from build123d import *

# Parameters (mm, degrees)
SKETCH1_W                  = 650
SKETCH1_H                  = 160
BOSS_EXTRUDE1_DEPTH        = 20
FILLET1_R                  = 10
F_11_0_11_DIAMETER_HOLE1_D = 11
F_7_0_7_DIAMETER_HOLE1_D   = 7
F_4_0_4_DIAMETER_HOLE1_D   = 4
M8_CLEARANCE_HOLE1_D       = 8.4


with BuildPart() as part:
    # Sketch1 → Boss-Extrude1 (new body)
    with BuildSketch(Plane(origin=(0, 0, 0), x_dir=(1, 0, 0), z_dir=(0, 1, 0))):
        with Locations((325, 80)):
            Rectangle(SKETCH1_W, SKETCH1_H)
    extrude(amount=BOSS_EXTRUDE1_DEPTH)

    # Fillet1
    fillet1_edges = [part.edges().sort_by_distance(p)[0] for p in [
        (0, 10, 0),
        (650, 10, 0),
        (650, 10, -160),
        (0, 10, -160),
    ]]
    fillet(fillet1_edges, radius=FILLET1_R)

    # Ø11.0 (11) Diameter Hole1 (through all)
    with Locations(Plane(origin=(0, 20, 0), x_dir=(1, 0, 0), z_dir=(0, 1, 0))):
        with Locations((72.352582635, 96.89911856), (261.667898073, 48.548804186), (487.756692049, 100.98506062), (567.432562216, 48.548804186), (292.312463521, 96.89911856)):
            Hole(F_11_0_11_DIAMETER_HOLE1_D / 2)

    # Ø7.0 (7) Diameter Hole1 (through all)
    with Locations(Plane(origin=(0, 20, 0), x_dir=(1, 0, 0), z_dir=(0, 1, 0))):
        with Locations((192.887873399, 100.304070277), (83.929418471, 36.97196835), (391.0560633, 71.702475858), (577.647417365, 117.32882886), (479.58480793, 43.10088144)):
            Hole(F_7_0_7_DIAMETER_HOLE1_D / 2)

    # Ø4.0 (4) Diameter Hole1 (through all)
    with Locations(Plane(origin=(0, 20, 0), x_dir=(1, 0, 0), z_dir=(0, 1, 0))):
        with Locations((178.58707619, 37.652958693), (151.347462458, 89.408224784), (353.601594419, 24.71414217), (403.31388948, 111.880906113), (540.192948484, 66.254553112), (87.007836042, 66.254553112)):
            Hole(F_4_0_4_DIAMETER_HOLE1_D / 2)

    # M8 Clearance Hole1 (through all)
    with Locations(Plane(origin=(0, 20, 0), x_dir=(1, 0, 0), z_dir=(0, 1, 0))):
        with Locations((625, 80), (25, 80)):
            Hole(M8_CLEARANCE_HOLE1_D / 2)


solid = part.part
Part model, mm, in its own coordinate system. Coordinates: 2 decimals unless noted, no trailing zeros. Use a Markdown table: item, result. Add a question column.
Q1. Pin check, flat tip, straight feed: P1, Ø12, axis at x = 278, z = -138.5, coming from the -Y side. Stop position of the tip, or through.
Q2. Probe L1, parallel to Z at x = 192, y = 13.75; L2, parallel to Z at x = 84, y = 14.5; L3, parallel to X at y = 15.5, z = -44. List the from-to ranges inside material, lowest first.
Q3. Mould opens along Z. For faces 1 (the flat face through (0, 10, -79)), 2 (the flat face through (321, 10, 0)), 3 (the cylindrical face through (493.25, 9.86, -101.23)), 4 (the flat face through (321, 10, -160)) say: +Z half, -Z half, draft (parallel to the pull), parting line (faces both ways), or undercut.
Worked out:
| question | item | result |
|---|---|---|
| 1 | P1 | stops at y = 0 |
| 2 | L1 | z = -160 to -103.69, -96.92 to 0 |
| 2 | L2 | z = -160 to -40.47, -33.47 to 0 |
| 2 | L3 | x = 0 to 258.58, 264.76 to 476.2, 482.97 to 564.34, 570.52 to 650 |
| 3 | face 1 | draft |
| 3 | face 2 | +Z half |
| 3 | face 3 | undercut |
| 3 | face 4 | -Z half |
